Can you work these out from the model? Positions are in its coordinate system, mm. A direction names the side the tool comes from. Coordinates: 2 decimals unless noted, no trailing zeros. Order: outer loops, then holes, each group sorted by start corner. A loop starts at its lowest first (then second) coordinate and runs counter-clockwise, first axis right, second up. Notation, with made-up numbers: (11, 36) - (44, 36) arc R16 ccw to (44, 62) - close; hole circle Ø11 at (75.5, 63.5). An arc over 180 degrees is marked (long way). Use a Markdown table: item, result. Add a question column.
(1) On a 3-axis mill with a long thin cutter (end or side, diameter ignored), from which of +Z, -Z, +X, -X, +Y, -Y can I reach the whole of each face in a straight line? I mean faces 5 (the cylindrical face through (44.166, 8.746, -1.479)), 6 (the flat face through (36.34, 19.34, 2.99)), 7 (the flat face through (39.5, 23.1, -2.9)), 8 (the flat face through (11.851, 19, -1)), 9 (the flat face through (12.4, 18, -0.8)). Say none if no direction works.
(2) I want a section at D-D (y = 15.85). List the corners of the cut face in (x, z) for me, and give its area (3 significant figures).
(3) For pin 1 Ø3 at (x, z) = (32, -3) entering from -Y; pin 2 Ø2 at (x, y) = (39.52, 8.95) entering from -Z; pin 3 Ø13 at (x, y) = (23.5, 16) entering from -Z; pin 4 Ø1.2 at (x, y) = (40.5, 23.5) entering from -Z, each with a flat end and sliding along its axis, tell me the tip position at first contact or that it passes through.
(4) We'd pull the mould along Y, two halves only. Please class faces 1 (the cylindrical face through (13.55, 18.285, -0.789)), 2 (the cylindrical face through (2, 42, 2)), 3 (the flat face through (24.78, 26.04, 2.99)), 4 (the flat face through (0, 22, 2)): pulls with the +Y half, pulls with the -Y half, needs draft (parallel to the pull), parting line crosses it, or undercut.
(5) I want a section at A-A (y = 8.95). List the corners of the cut face in (x, z) for me.
(6) I want a section at B-B (x = 33.02). List the corners of the cut face in (y, z) for me.
(7) If I drill on L1, parallel to Y at x = 39.52, z = -1.85; L2, parallel to X at y = 8.95, z = 2.25; L3, parallel to Y at x = 33.02, z = -1.05, over which ranges is the centre line in solid material (lowest first)? Write a range as [from, to].
(8) I want a section at C-C (z = 1). List the corners of the cut face in (x, y) for me.
Autodesk Inventor part; units mm, degrees
ref_plane "YZ Plane" through (0, 0, 0) normal (1, 0, 0) x (0, 1, 0)
ref_plane "XZ Plane" through (0, 0, 0) normal (0, 1, 0) x (-1, 0, 0)
ref_plane "XY Plane" through (0, 0, 0) normal (0, 0, 1) x (1, 0, 0)
sketch "Sketch1" plane through (0, 0, 0) normal (0, 0, 1) x (1, 0, 0)
  line L0 (0, 0) -> (45, 0)
  line L1 (45, 0) -> (45, 43)
  line L2 (45, 43) -> (0, 43)
  line L3 (0, 43) -> (0, 0)
  line L4 (13.851, 13.85) -> (35.351, 13.85)
  line L5 (35.351, 13.85) -> (35.351, 25.05)
  line L6 (35.351, 25.05) -> (13.851, 25.05)
  line L7 (13.851, 25.05) -> (13.851, 13.85)
  dimension "d0" = 45
  dimension "d1" = 43
  dimension "d2" = 21.5
  dimension "d3" = 11.2
  dimension "d4" = 9.649
  dimension "d16" = 17.95
extrude "Extrusion1" add sketch "Sketch1" along normal blind 4
fillet "Fillet1" radius 5 4 edges at (45, 43, 2) (45, 0, 2) (0, 43, 2) (0, 0, 2)
ref_plane "Work Plane1" through (0, 0, -2.5) normal (0, 0, -1) x (-1, 0, 0)
sketch "Sketch2" plane through (0, 0, 4) normal (0, 0, 1) x (1, 0, 0)
  circle A0 centre (14.02, 35.95) radius 1.4
  circle A1 centre (33.02, 35.95) radius 1.4
  line L0 (0, 43) -> (0, 0)
  line L1 (45, 0) -> (45, 43)
  line L2 (45, 43) -> (0, 43)
  circle A2 centre (7.52, 8.95) radius 1.4
  circle A3 centre (39.52, 8.95) radius 1.4
  line L3 (13.851, 13.85) -> (13.851, 25.05)
  line L4 (35.351, 13.85) -> (13.851, 13.85)
  line L5 (13.851, 25.05) -> (35.351, 25.05)
  dimension "d8" = 2.8
  dimension "d9" = 2.8
  dimension "d14" = 2.8
  dimension "d15" = 2.8
  dimension "d18" = 32
  dimension "d19" = 6.331
  dimension "d20" = 4.9
  dimension "d22" = 19
  dimension "d23" = 10.9
  dimension "d24" = 10.9
  dimension "d25" = 0.169
  dimension "d28" = 4.9
extrude "Extrusion2" cut sketch "Sketch2" against normal through all
sketch "Sketch3" plane through (0, 0, 0) normal (0, 0, -1) x (-1, 0, 0)
  circle A0 centre (-39.52, 8.95) radius 1.4
  circle A1 centre (-39.52, 8.95) radius 4.65
  circle A2 centre (-33.02, 35.95) radius 1.4
  circle A3 centre (-33.02, 35.95) radius 4.65
  circle A4 centre (-14.02, 35.95) radius 1.4
  circle A5 centre (-14.02, 35.95) radius 4.65
  circle A6 centre (-7.52, 8.95) radius 1.4
  circle A7 centre (-7.52, 8.95) radius 4.65
  circle A8 centre (-39.52, 8.95) radius 1.4
  circle A9 centre (-7.52, 8.95) radius 1.4
  circle A10 centre (-14.02, 35.95) radius 1.4
  circle A11 centre (-33.02, 35.95) radius 1.4
  point P0 (0, 0)
  dimension "d30" = 9.3
  dimension "d31" = 9.3
  dimension "d32" = 9.3
  dimension "d33" = 9.3
sketch "Sketch4" plane through (0, 0, -2.5) normal (0, 0, -1) x (-1, 0, 0)
  circle A0 centre (-39.52, 8.95) radius 1.4
  circle A1 centre (-7.52, 8.95) radius 1.4
  circle A2 centre (-14.02, 35.95) radius 1.4
  circle A3 centre (-33.02, 35.95) radius 1.4
  circle A4 centre (-33.02, 35.95) radius 2.1
  circle A5 centre (-14.02, 35.95) radius 2.1
  circle A6 centre (-7.52, 8.95) radius 2.1
  circle A7 centre (-39.52, 8.95) radius 2.1
  point P0 (0, 0)
  dimension "d35" = 4.2
  dimension "d36" = 4.2
  dimension "d37" = 4.2
  dimension "d38" = 4.2
ref_plane "Work Plane2" through (39.52, 8.95, -2.5) normal (0, 0, -1) x (-1, 0, 0)
ref_plane "Work Plane3" through (7.52, 8.95, -2.5) normal (0, 0, -1) x (-1, 0, 0)
sketch "Sketch6" plane through (7.52, 8.95, -2.5) normal (0, 0, -1) x (-1, 0, 0)
  circle A0 centre (0, 0) radius 1.4
  circle A1 centre (0, 0) radius 2.15
  circle A2 centre (-32, 0) radius 1.4
  circle A3 centre (-32, 0) radius 2.15
  circle A4 centre (-25.5, 27) radius 1.4
  circle A5 centre (-25.5, 27) radius 2.15
  circle A6 centre (-6.5, 27) radius 2.15
  circle A7 centre (-6.5, 27) radius 1.4
  point P0 (7.52, -8.95)
chamfer "Chamfer1" distance 2 angle 45 4 edges at (24.601, 13.85, 4) (35.351, 19.45, 4) (24.601, 25.05, 4) (13.851, 19.45, 4)
sketch "Sketch7" plane through (0, 0, 0) normal (0, 0, -1) x (-1, 0, 0)
  line L0 (-13.851, 13.85) -> (-35.351, 13.85)
  line L1 (-13.851, 25.05) -> (-13.851, 13.85)
  line L2 (-35.351, 25.05) -> (-13.851, 25.05)
  line L3 (-35.351, 13.85) -> (-35.351, 25.05)
  line L4 (-12.851, 18) -> (-11.851, 18)
  line L5 (-11.851, 18) -> (-11.851, 20.9)
  line L6 (-11.851, 20.9) -> (-12.851, 20.9)
  line L7 (-13.851, 19.9) -> (-13.851, 19)
  arc A0 (-13.851, 19) -> (-12.851, 18) centre (-12.851, 19) ccw
  arc A1 (-12.851, 20.9) -> (-13.851, 19.9) centre (-12.851, 19.9) ccw
  circle A2 centre (-36.864, 19.438) radius 0.75
  circle A3 centre (-39.5, 23.05) radius 0.65
  circle A4 centre (-9.3, 15.85) radius 0.65
  circle A5 centre (-9.3, 15.85) radius 2
  circle A6 centre (-39.5, 23.05) radius 2
  point P0 (0, 0)
  point P1 (-13.851, 18)
  point P2 (-13.851, 20.9)
  dimension "d70" = 2
  dimension "d71" = 2.9
  dimension "d72" = 4.15
  dimension "d73" = 1
  dimension "d74" = 1.5
  dimension "d75" = 1.513
  dimension "d76" = 5.588
  dimension "d77" = 4.149
  dimension "d78" = 1.3
  dimension "d79" = 2
  dimension "d80" = 1.3
  dimension "d81" = 4.551
  dimension "d82" = 2
  dimension "d87" = 4
  dimension "d88" = 4
extrude "Extrusion5" add sketch "Sketch7" along normal blind 1.6 contours L1 A1 L6 L5 L4 A0 | A2 | A5 | A6
extrude "Extrusion6" add sketch "Sketch7" along normal blind 2.9 contours A3 | A4
extrude "Extrusion7" add sketch "Sketch3" along normal blind 3
extrude "Extrusion9" add sketch "Sketch4" along normal blind 2.6
ref_plane "Work Plane4" through (11.851, 19.45, -3.6) normal (0, 1, 0) x (-1, 0, 0)
ref_plane "Work Plane5" through (24.601, 11.85, -8.75) normal (1, 0, 0) x (0, 1, 0)
properties part number "Cover_new"
Answers follow:
| question | item | result |
|---|---|---|
| 1 | face 5 | -Z |
| 1 | face 6 | +Z |
| 1 | face 7 | -Z, +X, -X, +Y |
| 1 | face 8 | -Z, -X |
| 1 | face 9 | -Z, +X, -X |
| 2 | outline | (0, 0) - (7.3, 0) - (7.3, -1.6) - (8.65, -1.6) - (8.65, -2.9) - (9.95, -2.9) - (9.95, -1.6) - (11.3, -1.6) - (11.3, 0) - (13.85, 0) - (13.85, 2) - (11.85, 4) - (0, 4) - close; (35.35, 0) - (45, 0) - (45, 4) - (37.35, 4) - (35.35, 2) - close |
| 2 | area | 98.1 mm² |
| 3 | pin 1 | stops at y = 31.3 |
| 3 | pin 2 | passes through |
| 3 | pin 3 | stops at z = 0 |
| 3 | pin 4 | stops at z = -2.9 |
| 4 | face 1 | pulls with the -Y half |
| 4 | face 2 | pulls with the +Y half |
| 4 | face 3 | undercut |
| 4 | face 4 | needs draft |
| 5 | outline | (0, 0) - (2.87, 0) - (2.87, -3) - (5.42, -3) - (5.42, -5.1) - (6.12, -5.1) - (6.12, 4) - (0, 4) - close; (8.92, -5.1) - (9.62, -5.1) - (9.62, -3) - (12.17, -3) - (12.17, 0) - (34.87, 0) - (34.87, -3) - (37.42, -3) - (37.42, -5.1) - (38.12, -5.1) - (38.12, 4) - (8.92, 4) - close; (40.92, -5.1) - (41.62, -5.1) - (41.62, -3) - (44.17, -3) - (44.17, 0) - (45, 0) - (45, 4) - (40.92, 4) - close |
| 6 | outline | (0, 0) - (13.85, 0) - (13.85, 2) - (11.85, 4) - (0, 4) - close; (25.05, 0) - (31.3, 0) - (31.3, -3) - (33.85, -3) - (33.85, -5.1) - (34.55, -5.1) - (34.55, 4) - (27.05, 4) - (25.05, 2) - close; (37.35, -5.1) - (38.05, -5.1) - (38.05, -3) - (40.6, -3) - (40.6, 0) - (43, 0) - (43, 4) - (37.35, 4) - close |
| 7 | L1 | y = [4.3, 7.55], [10.35, 13.6], [22.4, 23.7] |
| 7 | L2 | x = [0, 6.12], [8.92, 38.12], [40.92, 45] |
| 7 | L3 | y = [31.3, 34.55], [37.35, 40.6] |
| 8 | outline | (0, 5) arc R5 ccw to (5, 0) - (40, 0) arc R5 ccw to (45, 5) - (45, 38) arc R5 ccw to (40, 43) - (5, 43) arc R5 ccw to (0, 38) - close; hole circle Ø2.8 at (7.52, 8.95); hole circle Ø2.8 at (14.02, 35.95); hole (13.85, 13.85) - (35.35, 13.85) - (35.35, 25.05) - (13.85, 25.05) - close; hole circle Ø2.8 at (33.02, 35.95); hole circle Ø2.8 at (39.52, 8.95) |
